Autodesk Inventor part; units mm, degrees
ref_plane "YZ Plane" through (0, 0, 0) normal (1, 0, 0) x (0, 1, 0)
ref_plane "XZ Plane" through (0, 0, 0) normal (0, 1, 0) x (-1, 0, 0)
ref_plane "XY Plane" through (0, 0, 0) normal (0, 0, 1) x (1, 0, 0)
sketch "Sketch1" plane through (0, 0, 0) normal (0, 1, 0) x (-1, 0, 0)
  line L0 (-15, 6) -> (15, 6)
  line L1 (15, 6) -> (15, -6)
  line L2 (15, -6) -> (-15, -6)
  line L3 (-15, -6) -> (-15, 6)
  line L4 (-15, 6) -> (15, -6) construction
  line L5 (15, 6) -> (-15, -6) construction
  point P0 (0, 0)
  dimension "d0" = 12
  dimension "d1" = 30
extrude "Extrusion1" add sketch "Sketch1" along normal mid plane 2
sketch "Sketch2" plane through (-15, -1, 6) normal (-1, 0, 0) x (0, 0, 1)
  circle A0 centre (-6, 9) radius 1.5875
  circle A1 centre (-6, 9) radius 2.75
  line L0 (-8.5267, 10.0854) -> (-12, 2)
  line L1 (0, 0) -> (0, 2)
  line L2 (-12, 2) -> (0, 2)
  line L3 (0, 2) -> (-3.4733, 10.0854)
  point P0 (-6, 1)
  dimension "d4" = 3.175
  dimension "d5" = 5.5
  dimension "d6" = 7
extrude "Extrusion2" add sketch "Sketch2" against normal blind 4
mirror "Mirror1" about plane through (0, 0, 0) normal (1, 0, 0) of "Extrusion2"
sketch "Sketch5" plane through (15, -1, 6) normal (1, 0, 0) x (0, 0, -1)
  line L0 (8.5267, 10.0854) -> (12, 2)
  line L1 (12, 2) -> (8.5267, 10.0854)
  line L2 (0.9727, 4.2642) -> (0.4323, 3.0064)
  line L3 (0, 2) -> (3.4733, 10.0854)
  circle A0 centre (6, 9) radius 1.5875
  circle A1 centre (6, 9) radius 2.75 construction
  line L4 (6.7482, 5.2835) -> (10.0744, 6.4827)
  line L5 (0.4323, 3.0064) -> (10.0744, 6.4827)
  arc A2 (8.5267, 10.0854) -> (3.4733, 10.0854) centre (6, 9) ccw
  line L6 (9.679, 7.4031) -> (10.0744, 6.4827)
  line L7 (0.9727, 4.2642) -> (9.679, 7.4031)
  line L8 (12, 0) -> (0, 0)
  point P0 (6, 1)
  dimension "d23" = 1
  dimension "d24" = 3.0064
extrude "Extrusion5" add sketch "Sketch5" along normal blind 1 contours L0 L4 L5 L2 L7
mirror "Mirror2" about plane through (0, 0, 0) normal (1, 0, 0) of "Extrusion5"
sketch "Sketch6" plane through (0, 1, 0) normal (0, 1, 0) x (1, 0, 0)
  point P0 (0, 0)
  point P1 (0, 0)
hole "Hole1" at (0, 1, 0) direction (0, -1, 0) diameter 4.496 depth 5.692 tip angle 118
properties part number "EpoxyFiberMountBase"
Input: part model. Units: mm. Frame: model coordinates. A direction names the side the tool comes from. Coordinates: 2 decimals unless noted, no trailing zeros. Loops run counter-clockwise (first coordinate to the right, second up) from the corner with the lowest first, then second, coordinate; pieces in that order, holes last. Notation, with made-up numbers: (28, 54.5) - (81, 54.5) arc R18 ccw to (81, 77.5) - close; hole circle Ø2 at (-32, 83). An arc over 180 degrees is marked (long way). Answer in a Markdown table with one row per item. Add a question column.
Item 1: Access query for faces 1 (the flat face through (-15.493, 4.856, 0.613)), 2 (the flat face through (11, 5, 0)), 3 (the flat face through (15.49, 4.81, 0.74)). Directions: +Z, -Z, +X, -X, +Y, -Y. A direction counts if a zero-diameter tool reaches every point of the face in a straight line with its end or side. Return the directions, or none.
Item 2: Section query C-C on z = 0. Return the cut outline in (x, y).
Item 3: Contact query for flat-ended pins moving along their axis: P1, Ø6, axis at x = 0, z = 0, coming from the +Y side; P2, Ø3.5, axis at y = 8.5, z = -1, coming from the +X side; P3, Ø6, axis at y = 8, z = 1, coming from the -X side; P4, Ø1.9, axis at y = 4, z = -2.5, coming from the -X side. Output: stop coordinate, or through.
Item 4: Line query: line 1 along X through (y, z) = (-0.5, 0); line 2 along X through (y, z) = (3.75, -1.5); line 3 along Z through (x, y) = (0, 0.1). Output: solid intervals per line, ascending. Write a range as [from, to].
Item 5: Section query A-A on x = 0. Return the cut outline in (y, z), then the cut area to 3 significant figures.
Item 6: Section query B-B on y = 8. Return the cut outline in (x, z).
Item 7: Mould query, pull axis X, two halves, no side actions, for faces 4 (the flat face through (15, 1, 0)), 5 (the flat face through (0, -1, 3)), 6 (the cylindrical face through (1.37, -0.01, -1.78)). Classes: released by +X, released by -X, zero draft, split by the parting line, or undercut.
Item 8: Section query D-D on z = -3.25. Return the cut outline in (x, y), then the cut area to 3 significant figures.
Recorded:
| question | item | result |
|---|---|---|
| 1 | face 1 | +Z, -X, +Y |
| 1 | face 2 | +Z, -Z, +Y |
| 1 | face 3 | +Z, +X, +Y |
| 2 | outline | (-16, 4.01) - (-15, 4.01) - (-15, -1) - (-2.25, -1) - (-2.25, 1) - (-11, 1) - (-11, 6.41) - (-15, 6.41) - (-15, 5.08) - (-16, 5.08) - close; (-15, 9.59) - (-11, 9.59) - (-11, 10.75) - (-15, 10.75) - close; (2.25, -1) - (15, -1) - (15, 4.01) - (16, 4.01) - (16, 5.08) - (15, 5.08) - (15, 6.41) - (11, 6.41) - (11, 1) - (2.25, 1) - close; (11, 9.59) - (15, 9.59) - (15, 10.75) - (11, 10.75) - close |
| 3 | P1 | y = 1 |
| 3 | P2 | x = 15 |
| 3 | P3 | x = -15 |
| 3 | P4 | x = -16 |
| 4 | line 1 | [-15, -2.25], [2.25, 15] |
| 4 | line 2 | [-15, -11], [11, 15] |
| 4 | line 3 | [-6, -2.25], [2.25, 6] |
| 5 | outline | (-1, -6) - (1, -6) - (1, -2.25) - (-1, -2.25) - close; (-1, 2.25) - (1, 2.25) - (1, 6) - (-1, 6) - close |
| 5 | area | 15.0 mm^2 |
| 6 | outline | (-15, -2.99) - (-11, -2.99) - (-11, -1.59) - (-15, -1.59) - close; (-15, 1.59) - (-11, 1.59) - (-11, 2.99) - (-15, 2.99) - close; (11, -2.99) - (15, -2.99) - (15, -1.59) - (11, -1.59) - close; (11, 1.59) - (15, 1.59) - (15, 2.99) - (11, 2.99) - close |
| 7 | face 4 | released by +X |
| 7 | face 5 | zero draft |
| 7 | face 6 | undercut |
| 8 | outline | (-16, 5.19) - (-15, 5.19) - (-15, -1) - (15, -1) - (15, 5.19) - (16, 5.19) - (16, 6.25) - (15, 6.25) - (15, 7.4) - (11, 7.4) - (11, 1) - (-11, 1) - (-11, 7.4) - (-15, 7.4) - (-15, 6.25) - (-16, 6.25) - close |
| 8 | area | 113 mm^2 |
